The model under review builds one solid part; all positions refer to its coordinate system, in mm. Face numbers are marked on the shaded views. A direction names the side the tool comes from. Give positions to 0.01 mm unless a question says otherwise; leave off trailing zeros. Loops run counter-clockwise (first coordinate to the right, second up) from the corner with the lowest first, then second, coordinate; pieces in that order, holes last. Notation, with made-up numbers: M -5,89 L 47,89 A32 ccw 47,119 Z; hole C -13,-8 d1. An arc over 180 degrees is marked long. Return JSON: item names as keys, results as strings. Group by question number.
Autodesk Inventor part; units mm, degrees
ref_plane "YZ Plane" through (0, 0, 0) normal (1, 0, 0) x (0, 1, 0)
ref_plane "XZ Plane" through (0, 0, 0) normal (0, 1, 0) x (-1, 0, 0)
ref_plane "XY Plane" through (0, 0, 0) normal (0, 0, 1) x (1, 0, 0)
sketch "Эскиз4" plane through (0, 0, 0) normal (0, 1, 0) x (-1, 0, 0)
  line L0 (-10, -10) -> (10, -10)
  line L1 (10, -10) -> (10, 10)
  line L2 (10, 10) -> (-10, 10)
  line L3 (-10, 10) -> (-10, -10)
  line L4 (-10, -10) -> (10, 10) construction
  line L5 (10, -10) -> (-10, 10) construction
  line L6 (-9.25, -9.25) -> (9.25, -9.25)
  line L7 (9.25, -9.25) -> (9.25, 9.25)
  line L8 (9.25, 9.25) -> (-9.25, 9.25)
  line L9 (-9.25, 9.25) -> (-9.25, -9.25)
  line L10 (-9.25, -9.25) -> (9.25, 9.25) construction
  line L11 (9.25, -9.25) -> (-9.25, 9.25) construction
  point P0 (0, 0)
  dimension "d11" = 20
  dimension "d12" = 20
  dimension "d13" = 18.5
  dimension "d14" = 18.5
sketch "Эскиз5" plane through (0, 0, 0) normal (1, 0, 0) x (0, 1, 0)
  line L0 (0, 0) -> (63.5, -109.9852)
  line L1 (0, 0) -> (127, 0) construction
  dimension "d15" = 127
  dimension "d16" = 60
sweep "Сдвиг1" add profiles "Эскиз4" path "Эскиз5"
sketch "Эскиз6" plane through (10, 0, 10) normal (1, 0, 0) x (0, 0, -1)
  line L0 (109.9852, 63.5) -> (119.9852, 57.7265)
  line L1 (20, 0) -> (129.9852, 63.5)
  line L2 (109.9852, 63.5) -> (121.5322, 63.5) construction
  line L3 (119.9852, 57.7265) -> (129.9852, 63.5)
  line L4 (129.9852, 63.5) -> (109.9852, 63.5)
  line L5 (129.2352, 63.5) -> (110.7352, 63.5)
  point P0 (10, 0)
  dimension "d19" = 30
extrude "Выдавливание3" cut sketch "Эскиз6" against normal blind 127.0171
sketch "Эскиз7" plane through (10, 0, 10) normal (1, 0, 0) x (0, 0, -1)
  line L0 (0, 0) -> (109.9852, 63.5)
  line L1 (109.9852, 63.5) -> (109.9852, 51.953)
  line L2 (20, 0) -> (119.9852, 57.7265)
  line L3 (109.9852, 63.5) -> (119.9852, 57.7265)
  line L4 (109.9852, 51.953) -> (109.9852, 51.4136)
  line L5 (109.9852, 51.4136) -> (120.7731, 57.642)
  line L6 (20, 0) -> (119.9852, 57.7265)
  line L7 (119.9852, 57.7265) -> (120.7731, 57.2716)
  point P0 (10, 0)
  point P1 (120.4523, 57.4568)
extrude "Выдавливание4" cut sketch "Эскиз7" against normal blind 127.0171
properties part number "КРЫШАДЕТАЛЬXI"
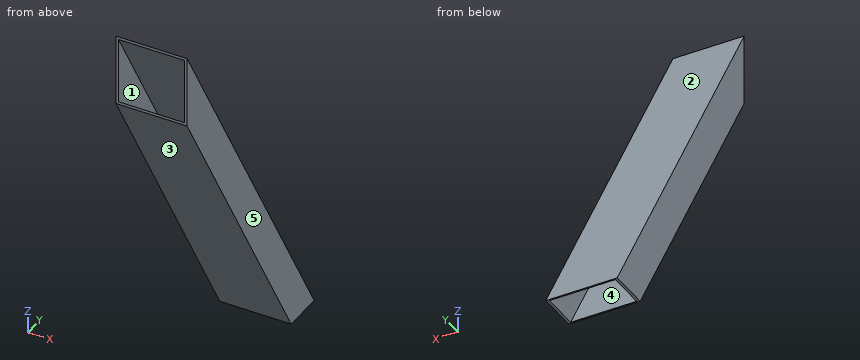
(1) For pin 1 (2 mm diameter, centred on x = 2, z = -5.5, fed in from -Y); pin 2 (10 mm diameter, centred on x = 0.5, z = -31.5, fed in from -Y); pin 3 (2 mm diameter, centred on x = -6, y = 55, fed in from -Z), all flat-tipped, find the tip position at first contact; note any pin that passes through.
(2) Add section B-B (z = -77). Write out the cut boundary in (x, y).
(3) Add section A-A (x = -2). Write out the cut boundary in (y, z), and give its area (3 significant figures).
(4) For probe 1 along X at (y, z) = (38, -68.5); probe 2 along Y at (x, z) = (-5.25, -90); probe 3 along Y at (x, z) = (8, -93.5), list the stretches that pass through material, from the lowest coordinate up.
(5) Mouldability with a two-part tool opening along Z and no side actions: class the marked faces 1, 2 and 3 as released by +Z, released by -Z, zero draft, split by the parting line, or undercut.
(6) Add section C-C (y = 13.5). Write out the cut boundary in (x, z).
(7) For the marked faces 4 and 5, list the 3-axis set-ups (+Z, -Z, +X, -X, +Y, -Y) from which the entire face can be reached by the end or side of a thin tool; tool diameter is ignored.
Verdict:
{
 "1": {"pin 1": "stops at y = 7.94", "pin 2": "stops at y = 9.53", "pin 3": "stops at z = -87.74"},
 "2": {"outline": "M -10,38.68 L 10,38.68 L 10,50.23 L -10,50.23 Z; hole M -9.25,39.12 L 9.25,39.12 L 9.25,49.8 L -9.25,49.8 Z"},
 "3": {"outline": "M 0,-10 L 51.95,-99.99 L 52.39,-99.99 L 0,-9.25 Z; M 0,9.25 L 63.07,-99.99 L 63.5,-99.99 L 0,10 Z", "area": "86.6 mm²"},
 "4": {"probe 1": "x = -10 to -9.25, 9.25 to 10", "probe 2": "y = 46.19 to 46.62, 57.3 to 57.74", "probe 3": "y = 48.21 to 48.64, 59.32 to 59.76"},
 "5": {"face 1": "undercut", "face 2": "released by +Z", "face 3": "released by -Z"},
 "6": {"outline": "M -10,-33.38 L 10,-33.38 L 10,-13.38 L -10,-13.38 Z; hole M -9.25,-32.63 L 9.25,-32.63 L 9.25,-14.13 L -9.25,-14.13 Z"},
 "7": {"face 4": "none", "face 5": "+Z, -Z, +X, +Y, -Y"}
}
